```python
from build123d import *

# Parameters (mm, degrees)
ESQUISSE1_W             = 30
ESQUISSE1_H             = 30
ESQUISSE1_W_2           = 20
ESQUISSE1_H_2           = 20
BOSS_EXTRU_1_DEPTH      = 30
ESQUISSE3_W             = 20
ESQUISSE3_H             = 25
ENL_V_MAT_EXTRU_1_DEPTH = 31
ESQUISSE4_W             = 20
ESQUISSE4_H             = 25
ENL_V_MAT_EXTRU_2_DEPTH = 31


with BuildPart() as part:
    # Esquisse1 → Boss.-Extru.1 (new body)
    with BuildSketch(Plane(origin=(0, 0, 0), x_dir=(1, 0, 0), z_dir=(0, 1, 0))):
        Rectangle(ESQUISSE1_W, ESQUISSE1_H)
        Rectangle(ESQUISSE1_W_2, ESQUISSE1_H_2, mode=Mode.SUBTRACT)
    extrude(amount=BOSS_EXTRU_1_DEPTH)

    # Esquisse3 → Enlèv. mat.-Extru.1 (cut, through all)
    with BuildSketch(Plane.XY.offset(15)):
        with Locations((0, 17.5)):
            Rectangle(ESQUISSE3_W, ESQUISSE3_H)
    extrude(amount=-ENL_V_MAT_EXTRU_1_DEPTH, mode=Mode.SUBTRACT)

    # Esquisse4 → Enlèv. mat.-Extru.2 (cut, through all)
    with BuildSketch(Plane.ZY.offset(15)):
        with Locations((0, 17.5)):
            Rectangle(ESQUISSE4_W, ESQUISSE4_H)
    extrude(amount=-ENL_V_MAT_EXTRU_2_DEPTH, mode=Mode.SUBTRACT)


solid = part.part
```
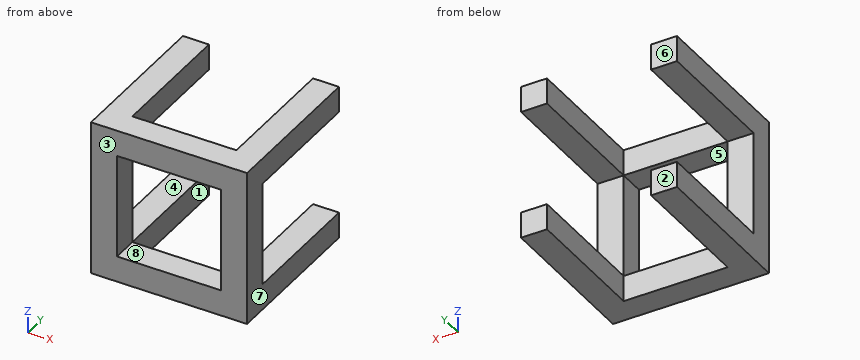
Geometry check sheet. Reference: the model listing, model coordinates, mm. Face numbers are marked on the shaded views. A direction names the side the tool comes from. Coordinates: 2 decimals unless noted, no trailing zeros. Write each loop counter-clockwise with the first axis right and the second up, starting at its lowest first coordinate (ties: lowest second). Pieces come first, ordered by that corner, then holes. Notation, with made-up numbers: M 75.5,75.25 L 119.5,75.25 A13 ccw 119.5,94.25 Z; hole C 37,-39 d2. An arc over 180 degrees is marked long. One line per item, written item: value. Start each with the question number.
(1) Sectioned sample at B-B, the plane x = -7. Enter the section's corners in (y, z).
(2) Scan lines: line 1 along Z through (x, y) = (13.25, 17.5); line 2 along Y through (x, z) = (9.25, -12.25). Record each from-to range of solid material in increasing order. Write a range as [from, to].
(3) Sectioned sample at A-A, the plane y = 26.5. Enter the section's corners in (x, z), and give its area (3 significant figures).
(4) Tool access check on the marked faces 1, 2, 3, 4 and 5. Record the directions out of +Z, -Z, +X, -X, +Y, -Y that give a thin tool (end or side, any length) a straight path to the whole face; none if there is none.
(5) Sectioned sample at D-D, the plane z = -0.5. Enter the section's corners in (x, y).
(6) Release check for a two-part mould opening along X. For the marked faces 6, 7 and 8 record: released by +X, released by -X, zero draft, split by the parting line, or undercut.
(7) Depth check by flat-ended pin: pin 1 (1.5 mm diameter, centred on x = 12.5, z = -3.5, fed in from +Y). Enter the tip coordinate at first touch or a pass-through.
(8) Sectioned sample at C-C, the plane y = 2. Enter the section's corners in (x, z).
Filled sheet:
1. outline: M 0,-15 L 5,-15 L 5,-10 L 0,-10 Z; M 0,10 L 5,10 L 5,15 L 0,15 Z
2. line 1: [-15, -10], [10, 15]
2. line 2: [0, 5]
3. outline: M -15,-15 L -10,-15 L -10,-10 L -15,-10 Z; M -15,10 L -10,10 L -10,15 L -15,15 Z; M 10,-15 L 15,-15 L 15,-10 L 10,-10 Z; M 10,10 L 15,10 L 15,15 L 10,15 Z
3. area: 100 mm²
4. face 1: +Z, -Z, +Y
4. face 2: +Z, -Z, +X, -X, +Y
4. face 3: +Z, -Z, +X, -X, -Y
4. face 4: +X, -X, +Y
4. face 5: +Y, -Y
5. outline: M -15,0 L -10,0 L -10,5 L -15,5 Z; M 10,0 L 15,0 L 15,5 L 10,5 Z
6. face 6: zero draft
6. face 7: released by +X
6. face 8: undercut
7. pin 1: y = 5
8. outline: M -15,-15 L 15,-15 L 15,15 L -15,15 Z; hole M -10,-10 L 10,-10 L 10,10 L -10,10 Z
